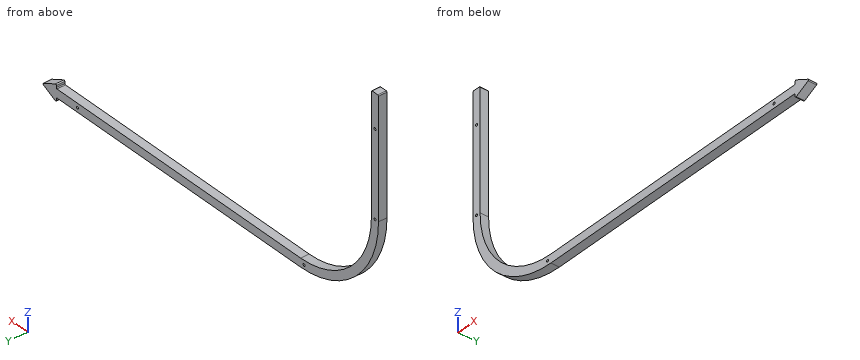
from build123d import *

# Parameters (mm, degrees)
SKETCH1_W               = 6.35
SKETCH1_H               = 88.9
SKETCH1_W_2             = 231.775
SKETCH1_H_2             = 6.35
SKETCH1_W_3             = 12.7
SKETCH1_H_3             = 12.7
BOSS_EXTRUDE1_DEPTH     = 6.35
CUT_EXTRUDE1_DEPTH      = 343.399866749
CUT_EXTRUDE1_DEPTH_BACK = 343.399866749
FILLET1_R               = 0.635
SKETCH3_R               = 0.889
CUT_EXTRUDE2_DEPTH      = 342.522840468


with BuildPart() as part:
    # Sketch1 → Boss-Extrude1 (new body)
    with BuildSketch(Plane(origin=(0, 0, 0), x_dir=(1, 0, 0), z_dir=(0, 1, 0))):
        with Locations((3.175, 44.45)):
            Rectangle(SKETCH1_W, SKETCH1_H)
        with BuildLine():
            ThreePointArc((0, 88.9), (20.458591334, 138.291408666), (69.85, 158.75))
            Line((69.85, 158.75), (69.85, 152.4))
            ThreePointArc((69.85, 152.4), (24.948719395, 133.801280605), (6.35, 88.9))
            Line((6.35, 88.9), (0, 88.9))
        make_face()
        with Locations((185.7375, 155.575)):
            Rectangle(SKETCH1_W_2, SKETCH1_H_2)
        with Locations((295.275, 155.575)):
            Rectangle(SKETCH1_W_3, SKETCH1_H_3)
    extrude(amount=BOSS_EXTRUDE1_DEPTH)

    # Sketch2 → Cut-Extrude1 (cut, two sides: drawn at the far end of the back side and taken through both)
    with BuildSketch(Plane(origin=(0, 6.35, 0), x_dir=(1, 0, 0), z_dir=(0, 1, 0)).offset(-CUT_EXTRUDE1_DEPTH_BACK)):
        Polygon((301.625, 161.925), (288.925, 161.925), (301.625, 155.575), align=None)
        Polygon((301.625, 149.225), (301.625, 155.575), (288.925, 149.225), align=None)
    extrude(amount=CUT_EXTRUDE1_DEPTH + CUT_EXTRUDE1_DEPTH_BACK, mode=Mode.SUBTRACT)

    # Fillet1
    fillet1_edges = [part.edges().sort_by_distance(p)[0] for p in [
        (0, 3.175, 0),
        (288.925, 3.175, -158.75),
        (288.925, 3.175, -152.4),
        (6.35, 3.175, 0),
        (288.925, 3.175, -161.925),
        (288.925, 3.175, -149.225),
        (301.625, 3.175, -155.575),
    ]]
    fillet(fillet1_edges, radius=FILLET1_R)

    # Sketch3 → Cut-Extrude2 (cut, through all)
    with BuildSketch(Plane(origin=(0, 6.35, 0), x_dir=(1, 0, 0), z_dir=(0, 1, 0))):
        with Locations(Location((3.175, 25.4, 0), (0, 0, 270))):
            Circle(SKETCH3_R)
        with Locations(Location((3.175, 88.9, 0), (0, 0, 270))):
            Circle(SKETCH3_R)
        with Locations(Location((66.802, 155.575, 0), (0, 0, 270))):
            Circle(SKETCH3_R)
        with Locations(Location((270.002, 155.575, 0), (0, 0, 270))):
            Circle(SKETCH3_R)
    extrude(amount=-CUT_EXTRUDE2_DEPTH, mode=Mode.SUBTRACT)


solid = part.part
The model under review builds one solid part; all positions refer to its coordinate system, in mm. Give positions to 0.01 mm unless a question says otherwise; leave off trailing zeros. Loops run counter-clockwise (first coordinate to the right, second up) from the corner with the lowest first, then second, coordinate; pieces in that order, holes last. Notation, with made-up numbers: (24.25, 68) -> (40.25, 68) arc R10 ccw to (40.25, 87) -> close; hole circle Ø5 at (19, -10). An arc over 180 degrees is marked (long way). Write each question's results on one line, items separated by ' | '.
1) For line 1 along X through (y, z) = (4.75, -25.4); line 2 along Z through (x, y) = (253, 0.75); line 3 along X through (y, z) = (6.25, -16), list the stretches that pass through material, from the lowest coordinate up. Write a range as from..to.
Conclusion:
line 1: x = 0..2.29, 4.06..6.35 | line 2: z = -158.75..-152.4 | line 3: x = 0..6.35
2) Take a section at A-A, the plane y = 2.5. Count the separate pieces of the cut face and the enclosed holes in it, plus the area to 3 significant figures.
Conclusion:
separate pieces: 1 | enclosed holes: 4 | area: 2,690 mm^2
3) Take a section at B-B, the plane z = -76.5. Give the boundary of the cut face in (x, y), plus the area to 3 significant figures.
Conclusion:
outline: (0, 0) -> (6.35, 0) -> (6.35, 6.35) -> (0, 6.35) -> close | area: 40.3 mm^2
4) Insertion check: pin 1 Ø1.6 at (x, z) = (3.175, -88.9) entering from +Y; pin 2 Ø1 at (y, z) = (1.5, -124) entering from -X; pin 3 Ø1.7 at (y, z) = (4, -160.5) entering from -X (3 decimals); pin 4 Ø1.9 at (x, y) = (206, 3) entering from +Z. Each pin has a flat end and moves straight along its axis. Give the tip position at first contact, or say it passes through.
Conclusion:
pin 1: passes through | pin 2: stops at x = 9.17 | pin 3: stops at x = 288.925 | pin 4: stops at z = -152.4
5) Take a section at C-C, the plane x = 212. Give the boundary of the cut face in (y, z).
Conclusion:
outline: (0, -158.75) -> (6.35, -158.75) -> (6.35, -152.4) -> (0, -152.4) -> close
